Geometry: final body of the model. Coordinates: model frame, mm. A direction names the side the tool comes from. Give positions to 0.01 mm unless a question says otherwise; leave off trailing zeros. Write each loop counter-clockwise with the first axis right and the second up, starting at its lowest first coordinate (ties: lowest second). Pieces come first, ordered by that corner, then holes. Notation, with made-up numbers: M -7.5,-26.5 L 26.5,-26.5 A11 ccw 26.5,-6.5 Z; hole C 40,20.25 d5. An arc over 180 degrees is marked long. Use one line per item in the form item = value. Start each with the question number.
Item 1: Access query for faces 1 (the flat face through (29, 50.8, 20)), 2 (the flat face through (-1, -7, -76.2)), 3 (the cylindrical face through (-0.95, 101.07, -28.43)), 4 (the flat face through (-29, 50.8, 20)), 5 (the flat face through (29, 50.8, -71)). Directions: +Z, -Z, +X, -X, +Y, -Y. A direction counts if a zero-diameter tool reaches every point of the face in a straight line with its end or side. Return the directions, or none.
Item 2: Material intervals for line 1 along Z through (x, y) = (1, 23.5); line 2 along Y through (x, z) = (-24, -38); line 3 along Y through (x, z) = (-3.5, -49), sorted ascending. Write a range as from..to.
Item 3: Contact query for flat-ended pins moving along their axis: P1, Ø6, axis at x = 4.5, y = 53, coming from the -Z side; P2, Ø4, axis at x = -16, z = 7.5, coming from the -Y side; P3, Ø2, axis at x = 19.5, z = -63.5, coming from the -Y side; P4, Ø19, axis at x = 18.5, z = -67, coming from the +Y side. Output: stop coordinate, or through.
Item 4: Section query B-B on y = 0. Return loops of the section in (x, z), then the cut area to 3 significant figures.
Item 5: Section query A-A on z = -25.4. Return loops of the section in (x, y) (3 decimals), then the cut area to 3 significant figures.
Item 6: Section query D-D on y = -47. Return loops of the section in (x, z), then the cut area to 3 significant figures.
Item 7: Pull-direction query (Y, two-part tool) for faces 6 (the flat face through (-1, -6, 25.4)), 7 (the cylindrical face through (2.93, 5.634, -25.044)), 8 (the flat face through (-29, 50.8, -71)); classes: released by +Y, released by -Y, zero draft, split by the parting line, or undercut.
Item 8: Section query C-C on x = -45.5. Return loops of the section in (y, z), then the cut area to 3 significant figures.
from build123d import *

# Parameters (mm, degrees)
SKETCH2_R           = 63.5
BOSS_EXTRUDE1_DEPTH = 25.4
SKETCH3_R           = 6.35
BOSS_EXTRUDE2_DEPTH = 50.8
BOSS_EXTRUDE3_START = 25.4
SKETCH4_R           = 63.5
BOSS_EXTRUDE3_DEPTH = 25.4
CUT_EXTRUDE1_START  = 76.2
SKETCH5_W           = 127
SKETCH5_H           = 101.6
CUT_EXTRUDE1_DEPTH  = 25.4
SKETCH6_R           = 50.8
BOSS_EXTRUDE4_DEPTH = 12.7
SKETCH7_R           = 3.175
BOSS_EXTRUDE5_DEPTH = 76.2


with BuildPart() as part:
    # Sketch2 → Boss-Extrude1 (new body)
    with BuildSketch(Plane.XY):
        Circle(SKETCH2_R)
    extrude(amount=BOSS_EXTRUDE1_DEPTH)

    # Sketch3 → Boss-Extrude2 (add)
    with BuildSketch(Plane(origin=(0, 0, 0), x_dir=(-1, 0, 0), z_dir=(0, 0, -1))):
        with Locations(Location((0, 0, 0), (0, 0, 180))):
            Circle(SKETCH3_R)
    extrude(amount=BOSS_EXTRUDE2_DEPTH)

    # Sketch4 → Boss-Extrude3 (add)
    with BuildSketch(Plane(origin=(0, 0, -50.8), x_dir=(-1, 0, 0), z_dir=(0, 0, -1)).offset(BOSS_EXTRUDE3_START)):
        with Locations(Location((0, 0, 0), (0, 0, 180))):
            Circle(SKETCH4_R)
    extrude(amount=-BOSS_EXTRUDE3_DEPTH)

    # Sketch5 → Cut-Extrude1 (cut)
    with BuildSketch(Plane(origin=(0, 0, 0), x_dir=(1, 0, 0), z_dir=(0, 1, 0)).offset(CUT_EXTRUDE1_START)):
        with Locations((0, 25.4)):
            Rectangle(SKETCH5_W, SKETCH5_H)
    extrude(amount=-CUT_EXTRUDE1_DEPTH, mode=Mode.SUBTRACT)

    # Sketch6 → Boss-Extrude4 (add)
    with BuildSketch(Plane(origin=(0, 50.8, 0), x_dir=(1, 0, 0), z_dir=(0, 1, 0))):
        with Locations(Location((0, 25.4, 0), (0, 0, 270))):
            Circle(SKETCH6_R)
    extrude(amount=BOSS_EXTRUDE4_DEPTH)

    # Sketch7 → Boss-Extrude5 (add)
    with BuildSketch(Plane(origin=(0, 63.5, 0), x_dir=(1, 0, 0), z_dir=(0, 1, 0))):
        with Locations(Location((0, 25.4, 0), (0, 0, 90))):
            Circle(SKETCH7_R)
    extrude(amount=BOSS_EXTRUDE5_DEPTH)


solid = part.part
Answer sheet:
q1.face_1 = +Z, +X, +Y
q1.face_2 = -Z, +X, -X, +Y, -Y
q1.face_3 = +Y
q1.face_4 = +Z, -X, +Y
q1.face_5 = -Z, +X, +Y
q2.line_1 = -76.2..-50.8, 0..25.4
q2.line_2 = 50.8..63.5
q2.line_3 = -5.3..5.3, 50.8..63.5
q3.P1 = -76.2
q3.P2 = -61.94
q3.P3 = -60.75
q3.P4 = 63.5
q4.outline = M -63.5,-76.2 L 63.5,-76.2 L 63.5,-50.8 L 6.35,-50.8 L 6.35,0 L 63.5,0 L 63.5,25.4 L -63.5,25.4 L -63.5,0 L -6.35,0 L -6.35,-50.8 L -63.5,-50.8 Z
q4.area = 7,100 mm2
q5.outline = M -50.8,50.8 L 50.8,50.8 L 50.8,63.5 L 3.175,63.5 L 3.175,139.7 L -3.175,139.7 L -3.175,63.5 L -50.8,63.5 Z; C 0,0 d12.7
q5.area = 1,900 mm2
q6.outline = M -42.7,-76.2 L 42.7,-76.2 L 42.7,-50.8 L -42.7,-50.8 Z; M -42.7,0 L 42.7,0 L 42.7,25.4 L -42.7,25.4 Z
q6.area = 4,340 mm2
q7.face_6 = zero draft
q7.face_7 = undercut
q7.face_8 = released by +Y
q8.outline = M -44.29,-76.2 L 44.29,-76.2 L 44.29,-50.8 L -44.29,-50.8 Z; M -44.29,0 L 44.29,0 L 44.29,25.4 L -44.29,25.4 Z; M 50.8,-47.99 L 63.5,-47.99 L 63.5,-2.81 L 50.8,-2.81 Z
q8.area = 5,070 mm2
